Check sheet for the modelled part. Datum: model origin and axes. Units: mm. Give positions to 0.01 mm unless a question says otherwise; leave off trailing zeros. Order: outer loops, then holes, each group sorted by start corner. A loop starts at its lowest first (then second) coordinate and runs counter-clockwise, first axis right, second up.
```python
from build123d import *

# Parameters (mm, degrees)
SKETCH1_W               = 190
SKETCH1_H               = 190
BOSS_EXTRUDE1_DEPTH     = 3
CUT_EXTRUDE2_DEPTH      = 135.383778783
CUT_EXTRUDE2_DEPTH_BACK = 3
SKETCH2_OUTSIDE_W       = 245.744
SKETCH2_OUTSIDE_H       = 245.744
SKETCH4_W               = 80
SKETCH4_H               = 12
CUT_EXTRUDE4_DEPTH      = 3
CUT_EXTRUDE5_DEPTH      = 3


with BuildPart() as part:
    # Sketch1 → Boss-Extrude1 (new body)
    with BuildSketch(Plane(origin=(0, 0, 0), x_dir=(1, 0, 0), z_dir=(0, 1, 0))):
        Rectangle(SKETCH1_W, SKETCH1_H)
    extrude(amount=BOSS_EXTRUDE1_DEPTH)

    # Sketch2 outside → Cut-Extrude2 (cut, two sides: drawn at the far end of the back side and taken through both)
    with BuildSketch(Plane(origin=(0, 3, 0), x_dir=(1, 0, 0), z_dir=(0, 1, 0)).offset(-CUT_EXTRUDE2_DEPTH_BACK)):
        Rectangle(SKETCH2_OUTSIDE_W, SKETCH2_OUTSIDE_H)
        Polygon((-95, -95), (-95, -70), (-92, -70), (-92, -25), (-95, -25), (-95, 25), (-92, 25), (-92, 70), (-95, 70), (-95, 95), (89, 95), (89, 70), (95, 70), (95, 25), (89, 25), (89, -25), (95, -25), (95, -70), (89, -70), (89, -95), align=None, mode=Mode.SUBTRACT)
    extrude(amount=CUT_EXTRUDE2_DEPTH + CUT_EXTRUDE2_DEPTH_BACK, mode=Mode.SUBTRACT)

    # Sketch4 → Cut-Extrude4 (cut)
    with BuildSketch(Plane(origin=(0, 3, 0), x_dir=(1, 0, 0), z_dir=(0, 1, 0))):
        with Locations((-45, 89)):
            Rectangle(SKETCH4_W, SKETCH4_H)
        with Locations((-45, -89)):
            Rectangle(SKETCH4_W, SKETCH4_H)
    extrude(amount=-CUT_EXTRUDE4_DEPTH, mode=Mode.SUBTRACT)

    # Sketch5 → Cut-Extrude5 (cut)
    with BuildSketch(Plane.XY.offset(95)):
        Polygon((50.678414624, 3), (50.692948093, 0), (19.039732141, 0), (19.039732141, 3), align=None)
    cut_extrude5 = extrude(amount=-CUT_EXTRUDE5_DEPTH, mode=Mode.SUBTRACT)

    # Mirror1: Cut-Extrude5 across plane
    add(cut_extrude5.mirror(Plane.XY), mode=Mode.SUBTRACT)


solid = part.part
```
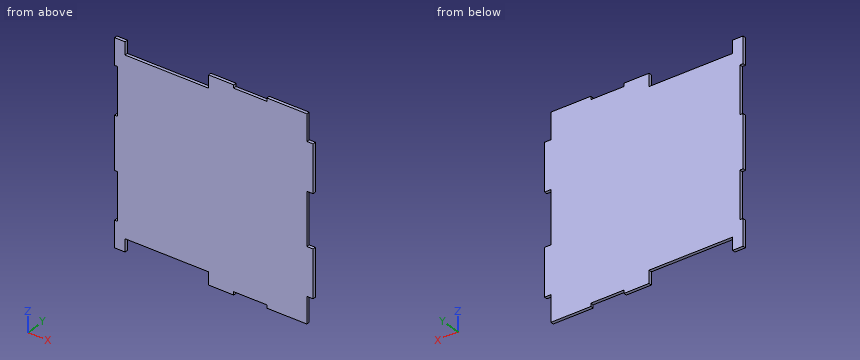
(1) Material ranges on L1, parallel to Z at x = -47, y = 1.6; L2, parallel to X at y = 2.65, z = -72; L3, parallel to Z at x = 42.5, y = 1.4, recorded low to high.
Response values:
L1: z = -83 to 83
L2: x = -95 to 89
L3: z = -92 to 92
(2) Gauge pin test, flat ends, axial feed: pin 1 Ø1 at (x, y) = (-23.5, 1.5) entering from +Z; pin 2 Ø1.5 at (y, z) = (1, 85) entering from +X; pin 3 Ø12 at (x, z) = (-30.5, 73) entering from -Y; pin 4 Ø0.9 at (y, z) = (1.5, -52) entering from -X. Record the tip position at first contact, or that the pin passes through.
Response values:
pin 1: stops at z = 83
pin 2: stops at x = 89
pin 3: stops at y = 0
pin 4: stops at x = -92
(3) Cross-section at A-A on z = -19.5. Enter the section's corners in (x, y), then the cut area to 3 significant figures.
Response values:
outline: (-95, 0) - (89, 0) - (89, 3) - (-95, 3) - close
area: 552 mm2
(4) Cross-section at B-B on x = -30.5. Enter the section's corners in (y, z).
Response values:
outline: (0, -83) - (3, -83) - (3, 83) - (0, 83) - close
